Source: CAD feature listing. Evaluate the final solid. Frame: model axes, mm. Face numbers are marked on the shaded views. A direction names the side the tool comes from. Give positions to 0.01 mm unless a question says otherwise; leave off trailing zeros. Write each loop counter-clockwise with the first axis right and the second up, starting at its lowest first coordinate (ties: lowest second). Pieces come first, ordered by that corner, then holes.
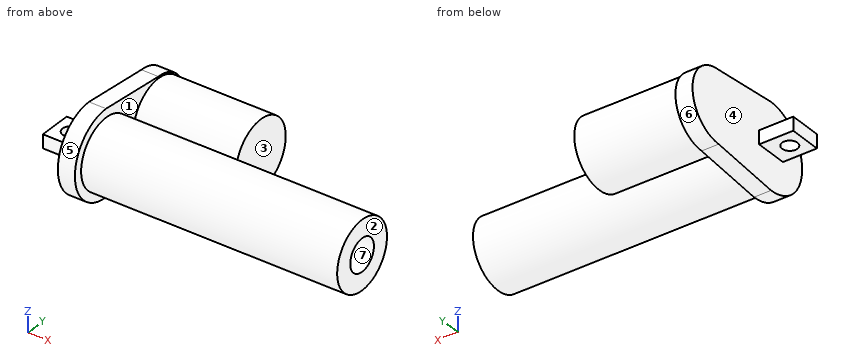
```python
from build123d import *

# Parameters (mm, degrees)
BOSS_EXTRUDE1_DEPTH = 10
BOSS_EXTRUDE2_DEPTH = 20
SKETCH3_R           = 4.5
CUT_EXTRUDE1_DEPTH  = 73.18032973
SKETCH5_R           = 20
BOSS_EXTRUDE4_DEPTH = 150
BOSS_EXTRUDE5_DEPTH = 60
SKETCH7_R           = 9.5
CUT_EXTRUDE2_DEPTH  = 150


with BuildPart() as part:
    # Sketch1 → Boss-Extrude1 (new body)
    with BuildSketch(Plane(origin=(0, 0, 0), x_dir=(0, 0, -1), z_dir=(1, 0, 0))):
        with BuildLine():
            Line((-21, 42), (-25, 0))
            ThreePointArc((-25, 0), (0, -25), (25, 0))
            Line((25, 0), (21, 42))
            ThreePointArc((21, 42), (0, 63), (-21, 42))
        make_face()
    extrude(amount=BOSS_EXTRUDE1_DEPTH)

    # Sketch2 → Boss-Extrude2 (add)
    with BuildSketch(Plane.ZY):
        Polygon((0, 9.5), (-4, 9.5), (-4, -9.5), (4, -9.5), (4, 9.5), align=None)
    extrude(amount=BOSS_EXTRUDE2_DEPTH)

    # Sketch3 → Cut-Extrude1 (cut, through all)
    with BuildSketch(Plane(origin=(0, 0, -4), x_dir=(-1, 0, 0), z_dir=(0, 0, -1))):
        with Locations(Location((11, 0, 0), (0, 0, 90))):
            Circle(SKETCH3_R)
    extrude(amount=-CUT_EXTRUDE1_DEPTH, mode=Mode.SUBTRACT)

    # Sketch5 → Boss-Extrude4 (add)
    with BuildSketch(Plane(origin=(10, 0, 0), x_dir=(0, 0, -1), z_dir=(1, 0, 0))):
        Circle(SKETCH5_R)
    extrude(amount=BOSS_EXTRUDE4_DEPTH)

    # Sketch6 → Boss-Extrude5 (add)
    with BuildSketch(Plane(origin=(10, 0, 0), x_dir=(0, 0, -1), z_dir=(1, 0, 0))):
        with BuildLine():
            ThreePointArc((-20, 42), (0, 22), (20, 42))
            Line((20, 42), (-20, 42))
        make_face()
        with BuildLine():
            Line((-20, 42), (20, 42))
            ThreePointArc((20, 42), (0, 62), (-20, 42))
        make_face()
    extrude(amount=BOSS_EXTRUDE5_DEPTH)

    # Sketch7 → Cut-Extrude2 (cut)
    with BuildSketch(Plane(origin=(160, 0, 0), x_dir=(0, 0, -1), z_dir=(1, 0, 0))):
        Circle(SKETCH7_R)
    extrude(amount=-CUT_EXTRUDE2_DEPTH, mode=Mode.SUBTRACT)


solid = part.part
```
1. Access query for the marked faces 1, 2 and 3. Directions: +Z, -Z, +X, -X, +Y, -Y. A direction counts if a zero-diameter tool reaches every point of the face in a straight line with its end or side. Return the directions, or none.
2. Mould query, pull axis Y, two halves, no side actions, for the marked faces 4, 5, 6 and 7. Classes: +Y half, -Y half, draft (parallel to the pull), parting line (faces both ways), or undercut.
3. Cut plane D-D, the plane z = -7.5. Return the cut outline in (x, y).
4. Line query: L1, parallel to Y at x = 53.5, z = 0; L2, parallel to Y at x = 75, z = 0; L3, parallel to X at y = 0, z = -2. Output: solid intervals per line, ascending.
5. Contact query for flat-ended pins moving along their axis: P1, Ø12, axis at x = 93, z = 8, coming from the +Y side; P2, Ø1.5, axis at y = 6.5, z = 18, coming from the -X side; P3, Ø1, axis at y = -8.5, z = -19, coming from the +X side; P4, Ø5.5, axis at x = -11, y = 0, coming from the +Z side. Output: stop coordinate, or through.
6. Cut plane C-C, the plane y = 28.5. Return the cut outline in (x, z).
7. Cut plane B-B, the plane x = 64. Return the cut outline in (y, z).
8. Cut plane A-A, the plane z = 0. Return the cut outline in (x, y), then the cut area to 3 significant figures.
Response values:
1. face 1: +X
1. face 2: +Z, -Z, +X, +Y, -Y
1. face 3: +Z, -Z, +X, +Y
2. face 4: draft
2. face 5: -Y half
2. face 6: +Y half
2. face 7: undercut
3. outline: (0, -23.85) - (10, -23.85) - (10, -18.54) - (160, -18.54) - (160, -5.83) - (10, -5.83) - (10, 5.83) - (160, 5.83) - (160, 18.54) - (10, 18.54) - (10, 23.46) - (70, 23.46) - (70, 60.54) - (10, 60.54) - (10, 61.62) - (0, 61.62) - close
4. L1: y = -20 to -9.5, 9.5 to 20, 22 to 62
4. L2: y = -20 to -9.5, 9.5 to 20
4. L3: x = -20 to -15.5, -6.5 to 10
5. P1: stops at y = 19.9
5. P2: stops at x = 0
5. P3: stops at x = 10
5. P4: passes through
6. outline: (0, -22.29) - (10, -22.29) - (10, -14.76) - (70, -14.76) - (70, 14.76) - (10, 14.76) - (10, 22.29) - (0, 22.29) - close
7. outline: circle Ø40 at (0, 0); circle Ø40 at (42, 0); hole circle Ø19 at (0, 0)
8. outline: (-20, -9.5) - (0, -9.5) - (0, -25) - (10, -25) - (10, -20) - (160, -20) - (160, -9.5) - (10, -9.5) - (10, 9.5) - (160, 9.5) - (160, 20) - (10, 20) - (10, 22) - (70, 22) - (70, 62) - (10, 62) - (10, 63) - (0, 63) - (0, 9.5) - (-20, 9.5) - close; hole circle Ø9 at (-11, 0)
8. area: 6,750 mm2
